Autodesk Inventor part; units mm, degrees
ref_plane "YZ Plane" through (0, 0, 0) normal (1, 0, 0) x (0, 1, 0)
ref_plane "XZ Plane" through (0, 0, 0) normal (0, 1, 0) x (-1, 0, 0)
ref_plane "XY Plane" through (0, 0, 0) normal (0, 0, 1) x (1, 0, 0)
sketch "Sketch1" plane through (0, 0, 0) normal (0, 0, 1) x (1, 0, 0)
  line L0 (0, 0) -> (455.6125, 0)
  line L1 (455.6125, 0) -> (455.6125, 11.938)
  line L2 (455.6125, 11.938) -> (0, 11.938)
  line L3 (0, 11.938) -> (0, 0)
  dimension "d0" = 455.6125
  dimension "d1" = 11.938
extrude "Extrusion1" add sketch "Sketch1" along normal blind 76.2
sketch "Sketch2" plane through (0, 0, 76.2) normal (0, 0, 1) x (1, 0, 0)
  circle A0 centre (227.8126, 236.728) radius 228.6
  line L0 (455.6125, 11.938) -> (0, 11.938)
  line L1 (0, 11.938) -> (0, 0)
  dimension "d6" = 227.8126
  dimension "d7" = 224.79
  dimension "d8" = 457.2
extrude "Extrusion2" cut sketch "Sketch2" against normal through all
properties part number "Exhaust Frame Upper+Lower as-built" material "Wood (Oak)"
Geometry: final body of the model. Coordinates: model frame, mm. Coordinates: 2 decimals unless noted, no trailing zeros. Write each loop counter-clockwise with the first axis right and the second up, starting at its lowest first coordinate (ties: lowest second). Pieces come first, ordered by that corner, then holes. Notation, with made-up numbers: M 88.25,-31.5 L 135.25,-31.5 A13 ccw 135.25,-9.5 Z; hole C 62.25,-27 d2. An arc over 180 degrees is marked long. Answer as CSV lines item,"result". Start each with the question number.
Q1. Mould query, pull axis X, two halves, no side actions, for faces 1 (the flat face through (455.612, 6, 38)), 2 (the flat face through (364, 11.938, 38)), 3 (the flat face through (0, 6, 38)), 4 (the cylindrical face through (227.23, 8.13, 38.63)). Classes: released by +X, released by -X, zero draft, split by the parting line, or undercut.
Q2. Line query: line 1 (Y direction, x = 229, z = 67); line 2 (Y direction, x = 237.5, z = 5). Output: solid intervals per line, ascending. Write a range as from..to.
Q3. Cut plane A-A on z = 63. Return the cut outline in (x, y), then the cut area to 3 significant figures.
Q4. Cut plane B-B on x = 205.5. Return the cut outline in (y, z).
Findings below:
1,face 1,"released by +X"
1,face 2,"zero draft"
1,face 3,"released by -X"
1,face 4,"undercut"
2,line 1,"y = 0..8.13"
2,line 2,"y = 0..8.33"
3,outline,"M 0,0 L 455.61,0 L 455.61,11.94 L 269.37,11.94 A228.6 cw 186.25,11.94 L 0,11.94 Z"
3,area,"5,230 mm2"
4,outline,"M 0,0 L 9.22,0 L 9.22,76.2 L 0,76.2 Z"
